The drawing under review shows one solid part. Ordinate dimensions are in mm from its lowest x, y, z. A direction names the side the tool comes from. Round coordinates to 2 decimals unless told otherwise and drop trailing zeros. Loops run counter-clockwise (first coordinate to the right, second up) from the corner with the lowest first, then second, coordinate; pieces in that order, holes last. Notation, with made-up numbers: (34, 87) - (81, 87) arc R12 ccw to (81, 110) - close; hole circle Ø3 at (-4.75, 47). An arc over 180 degrees is marked (long way). Answer as CSV lines item,"result".
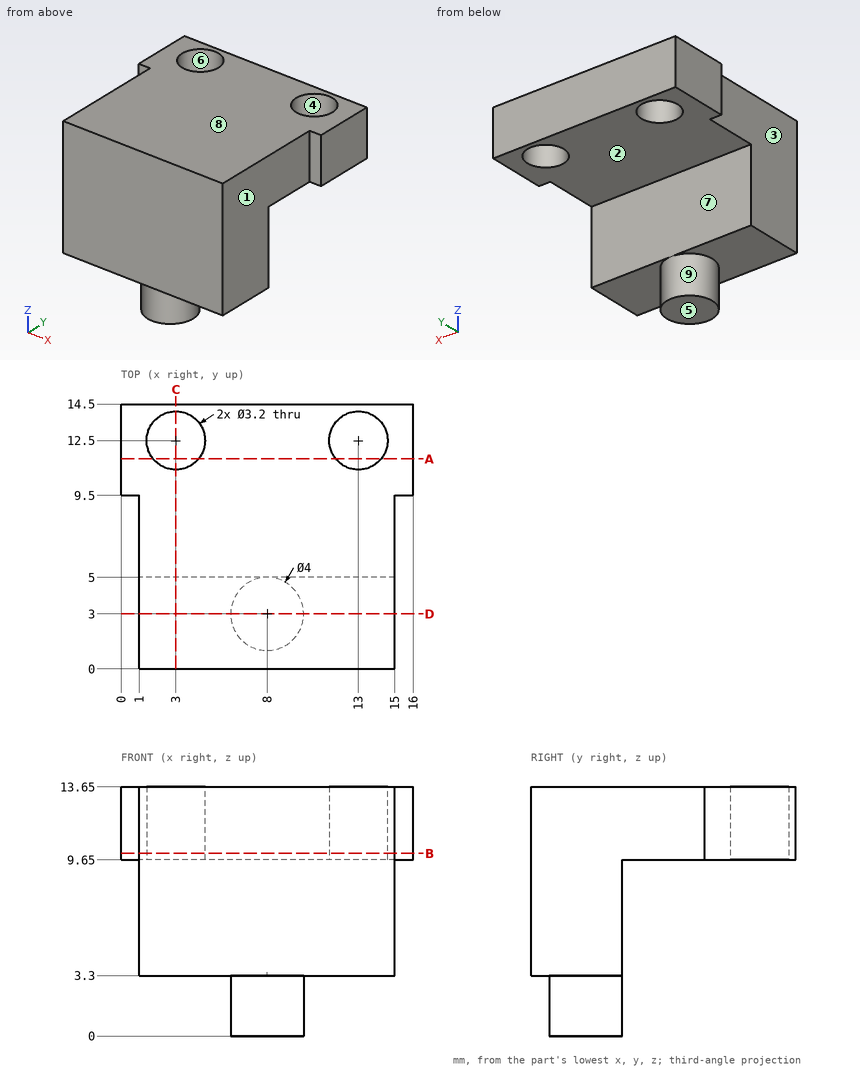
1. Take a section at D-D (y = 3). State the section outline as (x, z) points.
Numbers:
outline,"(1, 3.3) - (6, 3.3) - (6, 0) - (10, 0) - (10, 3.3) - (15, 3.3) - (15, 13.65) - (1, 13.65) - close"
2. Take a section at A-A (y = 11.5). State the section outline as (x, z) points, plus the area to 3 significant figures.
Numbers:
outline,"(0, 9.65) - (1.75, 9.65) - (1.75, 13.65) - (0, 13.65) - close; (4.25, 9.65) - (11.75, 9.65) - (11.75, 13.65) - (4.25, 13.65) - close; (14.25, 9.65) - (16, 9.65) - (16, 13.65) - (14.25, 13.65) - close"
area,"44.0 mm²"
3. Tool access review of the marked faces 1, 2, 3, 4 and 5: name each direction out of +Z, -Z, +X, -X, +Y, -Y from which nothing blocks a thin tool from reaching the whole face with its end or side.
Numbers:
face 1,"+Z, -Z, +X, -Y"
face 2,"-Z, +X, -X, +Y"
face 3,"+Z, -Z, -X, -Y"
face 4,"+Z, -Z"
face 5,"-Z, +X, -X, +Y, -Y"
4. Wall thickness on probe 1 along X at (y, z) = (12.5, 10.55); probe 2 along Y at (x, z) = (3, 12.45); probe 3 along Z at (x, y) = (8, 8): over which ranges is each line inside the solid? List them lowest first.
Numbers:
probe 1,"x = 0 to 1.4, 4.6 to 11.4, 14.6 to 16"
probe 2,"y = 0 to 10.9, 14.1 to 14.5"
probe 3,"z = 9.65 to 13.65"
5. Draft analysis for pull direction Y (two halves, no side actions). For the marked faces 6, 7, 8 and 9, state which applies: +Y half, -Y half, draft (parallel to the pull), parting line (faces both ways), or undercut.
Numbers:
face 6,"undercut"
face 7,"+Y half"
face 8,"draft"
face 9,"parting line"
6. Take a section at B-B (z = 10). State the section outline as (x, y) points, plus the area to 3 significant figures.
Numbers:
outline,"(0, 9.5) - (1, 9.5) - (1, 0) - (15, 0) - (15, 9.5) - (16, 9.5) - (16, 14.5) - (0, 14.5) - close; hole circle Ø3.2 at (3, 12.5); hole circle Ø3.2 at (13, 12.5)"
area,"197 mm²"
7. Clearance check with flat-ended pins moving along their axes: pin 1 (7.5 mm diameter, centred on x = 8.5, y = 11, fed in from -Z); pin 2 (2 mm diameter, centred on y = 3.5, z = 5.5, fed in from -X); pin 3 (4 mm diameter, centred on x = 4.5, z = 5.5, fed in from +Y). State where each tip first meets the part, or that it passes through.
Numbers:
pin 1,"stops at z = 9.65"
pin 2,"stops at x = 1"
pin 3,"stops at y = 5"
8. Take a section at C-C (x = 3). State the section outline as (y, z) points.
Numbers:
outline,"(0, 3.3) - (5, 3.3) - (5, 9.65) - (10.9, 9.65) - (10.9, 13.65) - (0, 13.65) - close; (14.1, 9.65) - (14.5, 9.65) - (14.5, 13.65) - (14.1, 13.65) - close"
